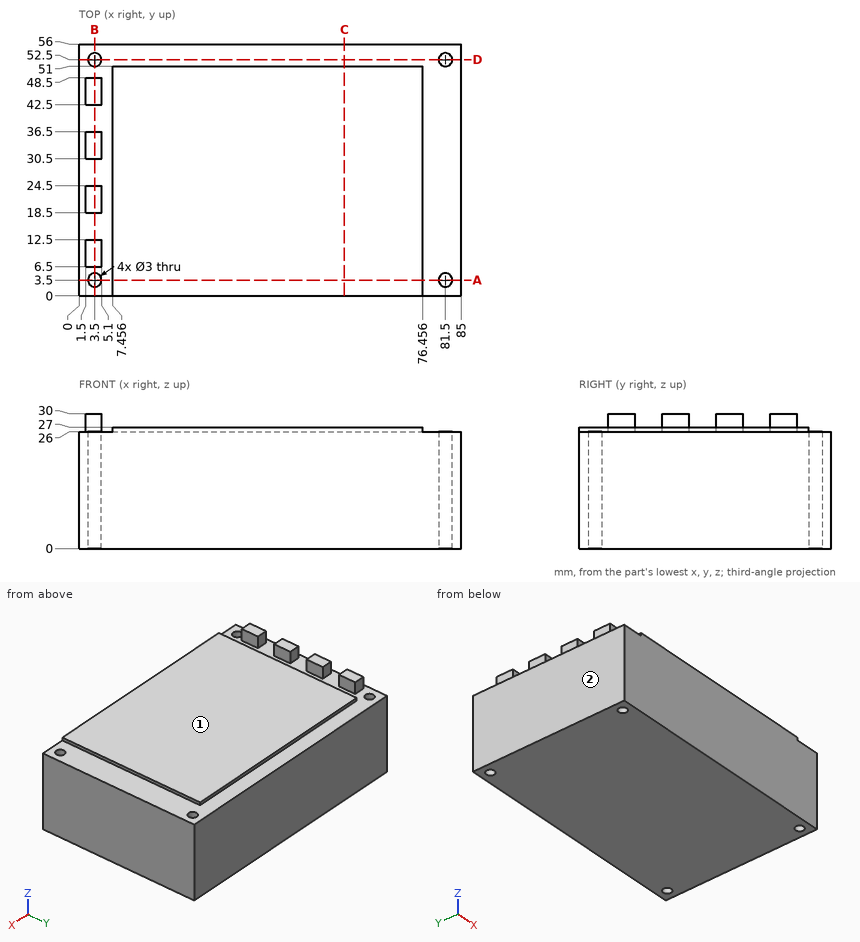
Print and shaded views of the part. All mm, measured from the part's lowest x, y and z. A direction names the side the tool comes from. Give positions to 0.01 mm unless a question says otherwise; leave off trailing zeros. Write each loop counter-clockwise with the first axis right and the second up, starting at its lowest first coordinate (ties: lowest second). Pieces come first, ordered by that corner, then holes. Notation, with made-up numbers: M 87,59 L 126,59 A19 cw 126,80 Z; hole C 87,-31.75 d9. An arc over 180 degrees is marked long. Use a Markdown table: item, result.
1) Cut at A-A (y = 3.5). List the corners of the cut face in (x, z).
Responses:
| item | result |
|---|---|
| outline | M 0,0 L 2,0 L 2,26 L 0,26 Z; M 5,0 L 80,0 L 80,26 L 76.46,26 L 76.46,27 L 7.46,27 L 7.46,26 L 5,26 Z; M 83,0 L 85,0 L 85,26 L 83,26 Z |
2) Drill centre lines: line 1 (Y direction, x = 3.5, z = 9.25); line 2 (Z direction, x = 42.5, y = 48); line 3 (Y direction, x = 29, z = 26.5). Where is each one in solid material? Low to high. Write a range as from..to.
Responses:
| item | result |
|---|---|
| line 1 | y = 0..2, 5..51, 54..56 |
| line 2 | z = 0..27 |
| line 3 | y = 0..51 |
3) Tool access for the marked faces 1 and 2: list every direction of +Z, -Z, +X, -X, +Y, -Y with a clear straight run to the whole face (end or side of a thin tool).
Responses:
| item | result |
|---|---|
| face 1 | +Z, +X, +Y, -Y |
| face 2 | +Z, -Z, -X, +Y, -Y |
4) Pin check, flat tips, straight feed: pin 1 (1.8 mm diameter, centred on x = 2.5, z = 27.5, fed in from -Y); pin 2 (1.5 mm diameter, centred on x = 47.5, y = 16.5, fed in from -Z); pin 3 (2.5 mm diameter, centred on x = 81.5, y = 52.5, fed in from -Z); pin 4 (1 mm diameter, centred on x = 39, y = 30.5, fed in from +Z). Stop position of each tip, or through.
Responses:
| item | result |
|---|---|
| pin 1 | stops at y = 6.5 |
| pin 2 | stops at z = 0 |
| pin 3 | passes through |
| pin 4 | stops at z = 27 |
5) Cut at D-D (y = 52.5). List the corners of the cut face in (x, z).
Responses:
| item | result |
|---|---|
| outline | M 0,0 L 2,0 L 2,26 L 0,26 Z; M 5,0 L 80,0 L 80,26 L 5,26 Z; M 83,0 L 85,0 L 85,26 L 83,26 Z |
6) Cut at C-C (x = 59). List the corners of the cut face in (y, z), and give its area (3 significant figures).
Responses:
| item | result |
|---|---|
| outline | M 0,0 L 56,0 L 56,26 L 51,26 L 51,27 L 0,27 Z |
| area | 1,510 mm2 |
7) Cut at B-B (x = 3.5). List the corners of the cut face in (y, z).
Responses:
| item | result |
|---|---|
| outline | M 0,0 L 2,0 L 2,26 L 0,26 Z; M 5,0 L 51,0 L 51,26 L 48.5,26 L 48.5,30 L 42.5,30 L 42.5,26 L 36.5,26 L 36.5,30 L 30.5,30 L 30.5,26 L 24.5,26 L 24.5,30 L 18.5,30 L 18.5,26 L 12.5,26 L 12.5,30 L 6.5,30 L 6.5,26 L 5,26 Z; M 54,0 L 56,0 L 56,26 L 54,26 Z |
